from build123d import *

# Parameters (mm, degrees)
SKETCH_R        = 4.5
SKETCH_R_2      = 1.5
PAD_DEPTH       = 9.4
SKETCH002_R     = 3.2
POCKET_DEPTH    = 3
SKETCH004_W     = 16.6
SKETCH004_H     = 6.4
POCKET002_DEPTH = 10
FILLET_R        = 0.4


with BuildPart() as part:
    # Sketch → Pad (new body)
    with BuildSketch(Plane.XY):
        with BuildLine():
            ThreePointArc((-16.650526, 21), (-18.950462, 18.950462), (-21, 16.650526))
            Line((-21, 16.650526), (-21, -16.650526))
            ThreePointArc((-21, -16.650526), (-18.950462, -18.950462), (-16.650526, -21))
            Line((-16.650526, -21), (16.650526, -21))
            ThreePointArc((16.650526, -21), (18.950462, -18.950462), (21, -16.650526))
            Line((21, -8.3), (21, -16.650526))
            Line((25.4, -8.3), (21, -8.3))
            Line((25.4, 8.3), (25.4, -8.3))
            Line((21, 8.3), (25.4, 8.3))
            Line((21, 16.650526), (21, 8.3))
            ThreePointArc((21, 16.650526), (18.950462, 18.950462), (16.650526, 21))
            Line((-16.650526, 21), (16.650526, 21))
        make_face()
        Circle(SKETCH_R, mode=Mode.SUBTRACT)
        with Locations((-15.5, 15.5)):
            Circle(SKETCH_R_2, mode=Mode.SUBTRACT)
        with Locations((15.5, 15.5)):
            Circle(SKETCH_R_2, mode=Mode.SUBTRACT)
        with Locations((15.5, -15.5)):
            Circle(SKETCH_R_2, mode=Mode.SUBTRACT)
        with Locations((-15.5, -15.5)):
            Circle(SKETCH_R_2, mode=Mode.SUBTRACT)
    extrude(amount=PAD_DEPTH)

    # Sketch002 → Pocket (cut)
    with BuildSketch(Plane.XY):
        with Locations((-15.5, 15.5)):
            Circle(SKETCH002_R)
        with Locations((15.5, 15.5)):
            Circle(SKETCH002_R)
        with Locations((15.5, -15.5)):
            Circle(SKETCH002_R)
        with Locations((-15.5, -15.5)):
            Circle(SKETCH002_R)
    extrude(amount=POCKET_DEPTH, mode=Mode.SUBTRACT)

    # Sketch004 → Pocket002 (cut)
    with BuildSketch(Plane.YZ.offset(26)):
        with Locations((0, 6.2)):
            Rectangle(SKETCH004_W, SKETCH004_H)
    extrude(amount=-POCKET002_DEPTH, mode=Mode.SUBTRACT)

    # Fillet
    fillet_edges = [part.edges().sort_by_distance(p)[0] for p in [
        (21, -8.3, 1.5),
        (21, 8.3, 1.5),
        (25.4, 8.3, 1.5),
        (25.4, -8.3, 1.5),
        (21, -16.650526, 4.7),
        (16.650526, -21, 4.7),
        (-16.650526, -21, 4.7),
        (-21, -16.650526, 4.7),
        (-21, 16.650526, 4.7),
        (-16.650526, 21, 4.7),
        (16.650526, 21, 4.7),
        (21, 16.650526, 4.7),
        (-18.7, 15.5, 0),
        (-18.7, -15.5, 0),
        (12.3, -15.5, 0),
        (12.3, 15.5, 0),
    ]]
    fillet(fillet_edges, radius=FILLET_R)


solid = part.part
Work out the finished part from the listing and answer in its coordinate system (mm). A direction names the side the tool comes from. Coordinates: 2 decimals unless noted, no trailing zeros. Loops run counter-clockwise (first coordinate to the right, second up) from the corner with the lowest first, then second, coordinate; pieces in that order, holes last. Notation, with made-up numbers: M 0.5,38 L 51.5,38 A17 cw 51.5,61 Z; hole C -2.5,-2.5 d11. An arc over 180 degrees is marked long. Answer in a Markdown table with one row per item. Add a question column.
1. Find section A-A, the plane x = -15.5. Write down the section's boundary in (y, z).
2. Find section D-D, the plane z = 4.75. Write down the section's boundary in (x, y).
3. Find section C-C, the plane x = 0. Write down the section's boundary in (y, z).
4. A tool of negligible diameter and unlimited length cuts with its end or side. For faces 1 (the flat face through (23, 8.3, 1)), 2 (the flat face through (-17, -16.2, 3)), 3 (the cylindrical face through (-0.59, 4.46, 4.63)), from which of +Z, -Z, +X, -X, +Y, -Y can it reach the whole face along a straight path? Write none if from no direction.
5. Flat-ended cylindrical pins translate along their axes: P1, Ø2.5, axis at x = 23, z = 1, coming from the -Y side; P2, Ø1.9, axis at x = 16, y = -17, coming from the -Z side; P3, Ø3, axis at y = 2, z = 6, coming from the +X side. Find the tip coordinate at first contact, or state that the pin passes through.
6. The mould has two halves that part along Y. Classify faces 4 (the flat face through (23, -8.3, 1)), 5 (the flat face through (16, 0, 6)), 6 (the flat face through (-21, 0, 5)), 7 (the cylindrical face through (-16.194, -18.624, 1.682)): pulls with the +Y half, pulls with the -Y half, needs draft (parallel to the pull), parting line crosses it, or undercut.
7. Consider L1, parallel to X at y = -15.5, z = 6; L2, parallel to Y at x = -15.5, z = 2.45. Determine where each line is inside the solid, lowest interval first.
Reported:
| question | item | result |
|---|---|---|
| 1 | outline | M -21,0 L -19.1,0 A0.4 ccw -18.7,0.4 L -18.7,3 L -17,3 L -17,9.4 L -21,9.4 Z; M -14,3 L -12.3,3 L -12.3,0.4 A0.4 ccw -11.9,0 L 11.9,0 A0.4 ccw 12.3,0.4 L 12.3,3 L 14,3 L 14,9.4 L -14,9.4 Z; M 17,3 L 18.7,3 L 18.7,0.4 A0.4 ccw 19.1,0 L 21,0 L 21,9.4 L 17,9.4 Z |
| 2 | outline | M -21,-16.51 A0.4 ccw -20.91,-16.76 A26.8 ccw -16.76,-20.91 A0.4 ccw -16.51,-21 L 16.51,-21 A0.4 ccw 16.76,-20.91 A26.8 ccw 20.91,-16.76 A0.4 ccw 21,-16.51 L 21,-8.3 L 16,-8.3 L 16,8.3 L 21,8.3 L 21,16.51 A0.4 ccw 20.91,16.76 A26.8 ccw 16.76,20.91 A0.4 ccw 16.51,21 L -16.51,21 A0.4 ccw -16.76,20.91 A26.8 ccw -20.91,16.76 A0.4 ccw -21,16.51 Z; hole C -15.5,-15.5 d3; hole C -15.5,15.5 d3; hole C 0,0 d9; hole C 15.5,-15.5 d3; hole C 15.5,15.5 d3 |
| 3 | outline | M -21,0 L -4.5,0 L -4.5,9.4 L -21,9.4 Z; M 4.5,0 L 21,0 L 21,9.4 L 4.5,9.4 Z |
| 4 | face 1 | +Z, -Z, +X, +Y |
| 4 | face 2 | -Z |
| 4 | face 3 | +Z, -Z |
| 5 | P1 | stops at y = -8.3 |
| 5 | P2 | stops at z = 3 |
| 5 | P3 | stops at x = 16 |
| 6 | face 4 | pulls with the -Y half |
| 6 | face 5 | undercut |
| 6 | face 6 | needs draft |
| 6 | face 7 | undercut |
| 7 | L1 | x = -21 to -17, -14 to 14, 17 to 21 |
| 7 | L2 | y = -21 to -18.7, -12.3 to 12.3, 18.7 to 21 |
